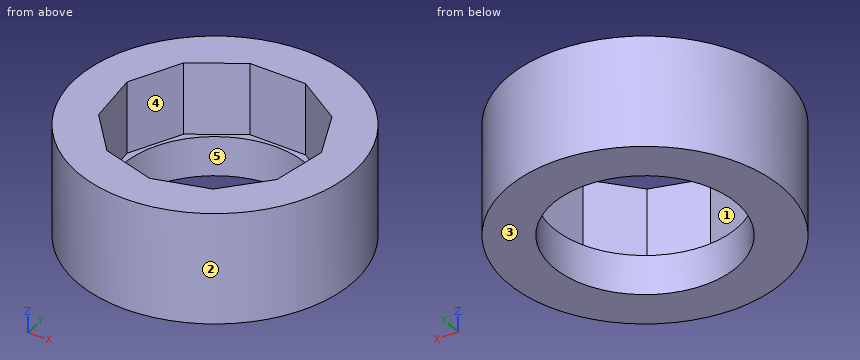
```python
from build123d import *

# Parameters (mm, degrees)
F0_R     = 39.9777863274
F1_DEPTH = 53.594
F3_DEPTH = 24.638
F4_DEPTH = 66.802
F5_R     = 26.7697870731
F6_DEPTH = 37.592
F7_DEPTH = 21.336


with BuildPart() as f1:
    # F0 (on Top) → F1 (new body)
    with BuildSketch(Plane.XY):
        Circle(F0_R)
    extrude(amount=F1_DEPTH)

    # F2 (on face) → F3 (join)
    with BuildSketch(Plane.XY.offset(53.594)):
        Polygon((-1.4570151686, -28.8758932938), (14.3857673972, -25.0796691189), (25.6611704593, -13.3208272032), (28.7893332138, 2.6672832291), (22.7770860886, 17.8085500823), (9.5332750655, 27.2957281135), (-6.7372834321, 28.1167053311), (-20.8688020433, 20.0108272692), (-28.3746234576, 5.5516529391), (-26.8717024097, -10.6701319731), (-16.8372057131, -23.5042253753), align=None)
    extrude(amount=F3_DEPTH)

    # F4 (cut): a face of the model
    f4_faces = [f1.faces().sort_by_distance(p)[0] for p in [
        (0, 0, 78.232),
    ]]
    extrude(f4_faces, amount=-F4_DEPTH, mode=Mode.SUBTRACT)

    # F5 (on face) → F6 (cut)
    with BuildSketch(Plane(origin=(0, 0, 0), x_dir=(1, 0, 0), z_dir=(0, 0, -1))):
        Circle(F5_R)
    extrude(amount=-F6_DEPTH, mode=Mode.SUBTRACT)

    # F7 (cut): a face of the model
    f7_faces = [f1.faces().sort_by_distance(p)[0] for p in [
        (-38.8470437751, 0, 53.594),
    ]]
    extrude(f7_faces, amount=-F7_DEPTH, mode=Mode.SUBTRACT)


solid = f1.part
```
Design review of the part built by this model. Coordinates are the model's own, in mm. Face numbers are marked on the shaded views. A direction names the side the tool comes from. Coordinates: 2 decimals unless noted, no trailing zeros. Loops run counter-clockwise (first coordinate to the right, second up) from the corner with the lowest first, then second, coordinate; pieces in that order, holes last.
Q1. Tool access review of the marked faces 4 and 5: name each direction out of +Z, -Z, +X, -X, +Y, -Y from which nothing blocks a thin tool from reaching the whole face with its end or side.
Reported:
face 4: +Z
face 5: +Z, -Z
Q2. The part is to be moulded in two halves that separate along Y. For the marked faces 1, 2 and 3, say which applies: +Y half, -Y half, draft (parallel to the pull), parting line (faces both ways), or undercut.
Reported:
face 1: undercut
face 2: parting line
face 3: draft
Q3. To check wall thickness, follow line 1 (Y direction, x = 0, z = 4); line 2 (Y direction, x = 15.5, z = 29); line 3 (Z direction, x = -28, y = 4). State the ranges of each line that lie inside material, in increasing order.
Reported:
line 1: y = -39.98 to -26.77, 26.77 to 39.98
line 2: y = -36.85 to -23.92, 23.02 to 36.85
line 3: z = 0 to 11.43
Q4. We need section B-B on y = 0. State the section outline as (x, z) points.
Reported:
outline: (-39.98, 0) - (-26.77, 0) - (-26.77, 11.43) - (-27.86, 11.43) - (-27.86, 32.26) - (-39.98, 32.26) - close; (26.77, 0) - (39.98, 0) - (39.98, 32.26) - (28.27, 32.26) - (28.27, 11.43) - (26.77, 11.43) - close
Q5. For pin 1 (2 mm diameter, centred on y = 17.5, z = 5, fed in from +X); pin 2 (6 mm diameter, centred on y = -8, z = 20, fed in from +X); pin 3 (5 mm diameter, centred on x = -26, y = -20.5, fed in from -Z); pin 4 (3 mm diameter, centred on x = 4.5, z = 8, fed in from +Y), all flat-tipped, find the tip position at first contact; note any pin that passes through.
Reported:
pin 1: stops at x = 36.41
pin 2: stops at x = 39.66
pin 3: stops at z = 0
pin 4: stops at y = 39.87
Q6. We need section C-C on x = 0. State the section outline as (y, z) points, and give its area (3 significant figures).
Reported:
outline: (-39.98, 0) - (-26.77, 0) - (-26.77, 11.43) - (-28.53, 11.43) - (-28.53, 32.26) - (-39.98, 32.26) - close; (26.77, 0) - (39.98, 0) - (39.98, 32.26) - (27.78, 32.26) - (27.78, 11.43) - (26.77, 11.43) - close
area: 795 mm2
Q7. We need section A-A on z = 17. State the section outline as (x, y) points.
Reported:
outline: circle Ø79.96 at (0, 0); hole (-28.37, 5.55) - (-26.87, -10.67) - (-16.84, -23.5) - (-1.46, -28.88) - (14.39, -25.08) - (25.66, -13.32) - (28.79, 2.67) - (22.78, 17.81) - (9.53, 27.3) - (-6.74, 28.12) - (-20.87, 20.01) - close
Q8. We need section D-D on z = 9. State the section outline as (x, y) points.
Reported:
outline: circle Ø79.96 at (0, 0); hole circle Ø53.54 at (0, 0)
